Here's the drawing with two shaded views (mm, measured from the low corner). I have some questions. A direction names the side the tool comes from. Round coordinates to 2 decimals unless told otherwise and drop trailing zeros. Order: outer loops, then holes, each group sorted by start corner. A loop starts at its lowest first (then second) coordinate and runs counter-clockwise, first axis right, second up.
Q1. If we section it at B-B (z = 2): Please give me the cut outline in (x, y).
Q2. Will these pins go through, and if not, where does the flat tip stop? P1, Ø3, axis at x = 51.5, z = 7, coming from the +Y side; P2, Ø4, axis at x = 16, z = 8.5, coming from the -Y side.
Q3. If we section it at A-A (x = 41): Please give me the cut outline in (y, z).
Q4. If I drill on line 1 (Z direction, x = 43, y = 18); line 2 (Y direction, x = 17, z = 6.25); line 3 (X direction, y = 7.5, z = 1.75), over which ranges is the centre line in solid material (lowest first)?
Q5. If we section it at D-D (z = 5.5): Please give me the cut outline in (x, y), plus the area to 3 significant figures.
Q6. If we section it at C-C (y = 7): Please give me the cut outline in (x, z).
Q7. For the marked faces 1, 2 and 3, which set-ups out of +Z, -Z, +X, -X, +Y, -Y let a thin tool reach every point of the face, with its end or its side?
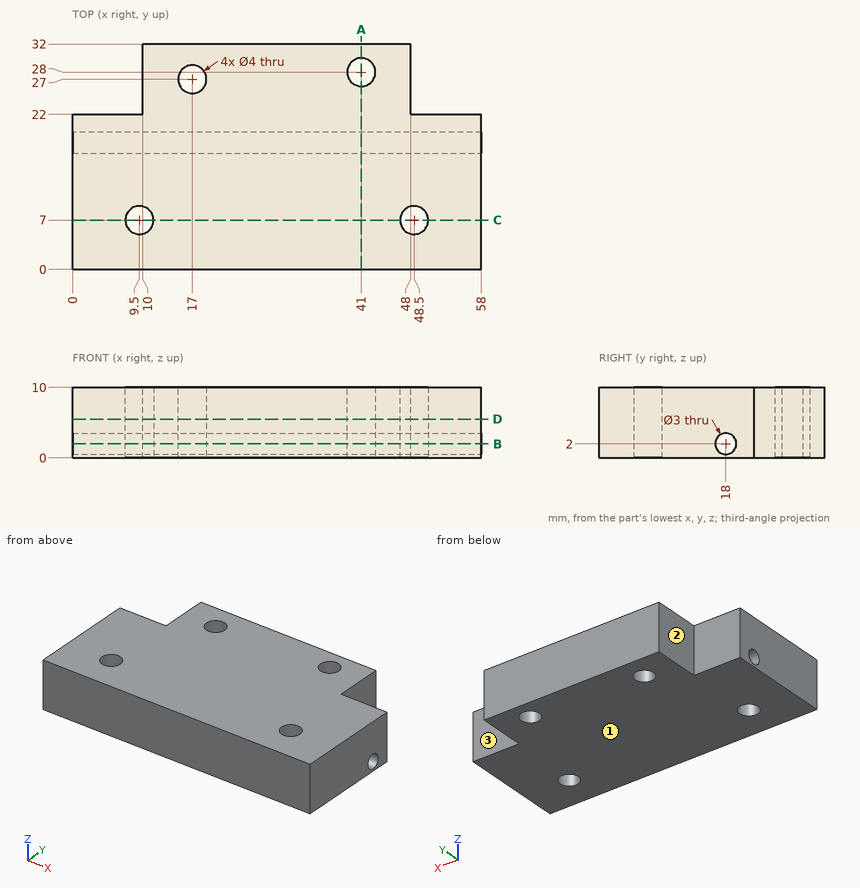
Solution:
1. outline: (0, 0) - (58, 0) - (58, 16.5) - (0, 16.5) - close; (0, 19.5) - (58, 19.5) - (58, 22) - (48, 22) - (48, 32) - (10, 32) - (10, 22) - (0, 22) - close; hole circle Ø4 at (9.5, 7); hole circle Ø4 at (17, 27); hole circle Ø4 at (41, 28); hole circle Ø4 at (48.5, 7)
2. P1: stops at y = 22
2. P2: stops at y = 0
3. outline: (0, 0) - (26, 0) - (26, 10) - (0, 10) - close; (30, 0) - (32, 0) - (32, 10) - (30, 10) - close; hole circle Ø3 at (18, 2)
4. line 1: z = 0 to 0.5, 3.5 to 10
4. line 2: y = 0 to 25, 29 to 32
4. line 3: x = 0 to 7.56, 11.44 to 46.56, 50.44 to 58
5. outline: (0, 0) - (58, 0) - (58, 22) - (48, 22) - (48, 32) - (10, 32) - (10, 22) - (0, 22) - close; hole circle Ø4 at (9.5, 7); hole circle Ø4 at (17, 27); hole circle Ø4 at (41, 28); hole circle Ø4 at (48.5, 7)
5. area: 1,610 mm2
6. outline: (0, 0) - (7.5, 0) - (7.5, 10) - (0, 10) - close; (11.5, 0) - (46.5, 0) - (46.5, 10) - (11.5, 10) - close; (50.5, 0) - (58, 0) - (58, 10) - (50.5, 10) - close
7. face 1: -Z, +X, -X, +Y, -Y
7. face 2: +Z, -Z, -X, +Y
7. face 3: +Z, -Z, +X, +Y
